Autodesk Inventor part; units mm, degrees
ref_plane "YZ Plane" through (0, 0, 0) normal (1, 0, 0) x (0, 1, 0)
ref_plane "XZ Plane" through (0, 0, 0) normal (0, 1, 0) x (-1, 0, 0)
ref_plane "XY Plane" through (0, 0, 0) normal (0, 0, 1) x (1, 0, 0)
sketch "Sketch1" plane through (0, 0, 0) normal (1, 0, 0) x (0, 1, 0)
  line L0 (0, 0) -> (0, 152.4)
  line L1 (0, 0) -> (330.2, 0)
  line L2 (0, 152.4) -> (342.9, 152.4)
  line L3 (342.9, 152.4) -> (342.9, 139.7) construction
  arc A0 (355.3918, 137.4098) -> (342.9, 152.4) centre (342.9, 139.7) ccw
  line L4 (330.2, 0) -> (355.3918, 137.4098)
  dimension "d0" = 152.4
  dimension "d1" = 330.2
  dimension "d2" = 342.9
  dimension "d3" = 12.7
extrude "Extrusion1" add sketch "Sketch1" along normal blind 1110.1916
properties part number "C" material "Granite, Cut, Polished"
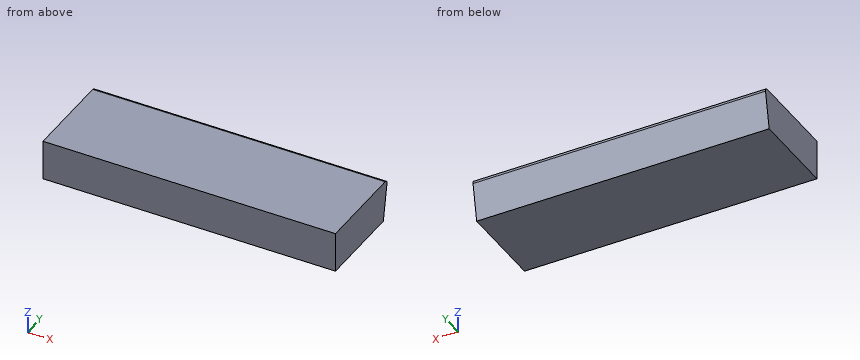
CAD build for the part. Positions are in the model's coordinates, mm. Round coordinates to 2 decimals unless told otherwise and drop trailing zeros. Write each loop counter-clockwise with the first axis right and the second up, starting at its lowest first coordinate (ties: lowest second). Pieces come first, ordered by that corner, then holes.
Item 1: Band-saw the part on A-A on x = 798. Write the cut outline in (y, z).
Filled in:
outline: (0, 0) - (330.2, 0) - (355.39, 137.41) arc R12.7 ccw to (342.9, 152.4) - (0, 152.4) - close
Item 2: Drill centre lines: L1, parallel to Y at x = 515, z = 140; L2, parallel to Y at x = 823.5, z = 132.5. Where is each one in solid material? Low to high.
Filled in:
L1: y = 0 to 355.6
L2: y = 0 to 354.49
Item 3: Drop flat-ended pins along their axis: pin 1 Ø2 at (x, z) = (591.5, 76.5) entering from -Y; pin 2 Ø5 at (x, z) = (364, 105) entering from +Y; pin 3 Ø1.5 at (x, z) = (539, 30.5) entering from +Y. Give the stop position or say it passes through.
Filled in:
pin 1: stops at y = 0
pin 2: stops at y = 349.91
pin 3: stops at y = 335.93
Item 4: Band-saw the part on B-B on z = 82.5. Write the cut outline in (x, y) (3 decimals).
Filled in:
outline: (0, 0) - (1110.192, 0) - (1110.192, 345.325) - (0, 345.325) - close
